```python
from build123d import *

# Parameters (mm, degrees)
SKETCH1_R                = 95.705
BOSS_EXTRUDE1_DEPTH      = 5
SKETCH2_W                = 15
SKETCH2_H                = 9.705675634
BOSS_EXTRUDE2_DEPTH      = 120
SKETCH3_R                = 95.705
SKETCH3_R_2              = 85.705
BOSS_EXTRUDE3_DEPTH      = 10
BOSS_EXTRUDE4_DEPTH      = 14.5
BOSS_EXTRUDE4_DEPTH_BACK = 14.5
SKETCH4_W                = 68.22
SKETCH4_H                = 26.18
SKETCH5_W                = 55
SKETCH5_H                = 20.8
CUT_EXTRUDE1_DEPTH       = 22.77
SKETCH6_W                = 40
SKETCH6_H                = 20.8
CUT_EXTRUDE2_DEPTH       = 5.77
SKETCH8_R                = 2.5
CUT_EXTRUDE3_DEPTH       = 5.77


with BuildPart() as part:
    # Sketch1 → Boss-Extrude1 (new body)
    with BuildSketch(Plane(origin=(0, 0, 0), x_dir=(1, 0, 0), z_dir=(0, 1, 0))):
        with Locations(Location((0, 0, 0), (0, 0, 94.494638706))):
            Circle(SKETCH1_R)
    extrude(amount=BOSS_EXTRUDE1_DEPTH)

    # Sketch2 → Boss-Extrude2 (add)
    with BuildSketch(Plane(origin=(0, 5, 0), x_dir=(1, 0, 0), z_dir=(0, 1, 0))):
        Polygon((83.827926187, 19.351377631), (93.058572244, 22.350596344), (88.423317328, 36.616444088), (79.192671271, 33.617225375), align=None)
        with Locations((0, 90.557837817)):
            Rectangle(SKETCH2_W, SKETCH2_H)
        Polygon((44.30850759, -73.745190895), (50.013360591, -81.597247425), (62.148615507, -72.780468641), (56.443762506, -64.928412111), align=None)
        Polygon((-56.443762506, -64.928412111), (-62.148615507, -72.780468641), (-50.013360591, -81.597247425), (-44.30850759, -73.745190895), align=None)
        Polygon((-79.192671271, 33.617225375), (-88.423317328, 36.616444088), (-93.058572244, 22.350596344), (-83.827926187, 19.351377631), align=None)
    extrude(amount=BOSS_EXTRUDE2_DEPTH)

    # Sketch3 → Boss-Extrude3 (add)
    with BuildSketch(Plane(origin=(0, 125, 0), x_dir=(1, 0, 0), z_dir=(0, 1, 0))):
        with Locations(Location((0, 0, 0), (0, 0, 94.494638706))):
            Circle(SKETCH3_R)
        Circle(SKETCH3_R_2, mode=Mode.SUBTRACT)
    extrude(amount=BOSS_EXTRUDE3_DEPTH)

    # Sketch4 → Boss-Extrude4 (add, two sides: drawn at the far end of the back side and taken through both)
    with BuildSketch(Plane(origin=(0, 130, 0), x_dir=(1, 0, 0), z_dir=(0, 1, 0)).offset(-BOSS_EXTRUDE4_DEPTH_BACK)):
        with Locations((-13.22, 84.54)):
            Rectangle(SKETCH4_W, SKETCH4_H)
    extrude(amount=BOSS_EXTRUDE4_DEPTH + BOSS_EXTRUDE4_DEPTH_BACK)

    # Sketch5 → Cut-Extrude1 (cut)
    with BuildSketch(Plane(origin=(0, 0, -97.63), x_dir=(-1, 0, 0), z_dir=(0, 0, -1))):
        with Locations((10, 130)):
            Rectangle(SKETCH5_W, SKETCH5_H)
    extrude(amount=-CUT_EXTRUDE1_DEPTH, mode=Mode.SUBTRACT)

    # Sketch6 → Cut-Extrude2 (cut)
    with BuildSketch(Plane(origin=(0, 0, -74.86), x_dir=(-1, 0, 0), z_dir=(0, 0, -1))):
        with Locations((10, 130)):
            Rectangle(SKETCH6_W, SKETCH6_H)
    extrude(amount=-CUT_EXTRUDE2_DEPTH, mode=Mode.SUBTRACT)

    # Sketch8 → Cut-Extrude3 (cut)
    with BuildSketch(Plane.XY.offset(90.705)):
        with Locations((0, 130)):
            Circle(SKETCH8_R)
    extrude(amount=-CUT_EXTRUDE3_DEPTH, mode=Mode.SUBTRACT)


solid = part.part
```
The listing builds one solid part. Answer for the finished solid, in the listing's coordinates (mm). A direction names the side the tool comes from. Round coordinates to 2 decimals unless told otherwise and drop trailing zeros. Write each loop counter-clockwise with the first axis right and the second up, starting at its lowest first coordinate (ties: lowest second). Pieces come first, ordered by that corner, then holes. Notation, with made-up numbers: (46.5, -24) -> (58.5, -24) arc R21 ccw to (58.5, 2) -> close; hole circle Ø1 at (10, 44). An arc over 180 degrees is marked (long way). Use CSV: the item, a comma, the result in double quotes. Start each with the question number.
(1) Which of the six approach directions +Z, -Z, +X, -X, +Y, -Y give full straight-line access (tool end or side, diameter ignored) to faces 1 (the face through (14, 130, -74.86)), 2 (the face through (0, 59, -85.705)), 3 (the face through (-7.5, 59, -90)), 4 (the face through (81.48, 64.16, -26.58)), 5 (the face through (88.38, 64.16, -20.83))?
(2) Section C-C on z = 0 is taken. Give the vertices of the cut face in (x, y) (3 decimals).
(3) Consider L1, parallel to X at y = 129, z = 0 (3 decimals); L2, parallel to Y at x = -80, z = -48; L3, parallel to Y at x = -18, z = 31.5. Determine where each line is inside the solid, lowest interval first. Write a range as from..to.
(4) Each of these flat-tipped pins is pushed along its axis until it touches: pin 1 (10.5 mm diameter, centred on y = 60.5, z = -91.5, fed in from -X); pin 2 (12 mm diameter, centred on x = 0, y = 85.5, fed in from +Z) (3 decimals); pin 3 (12 mm diameter, centred on x = -3, y = 74.5, fed in from -Z). Where does it stop, or does it pass through?
(5) Section B-B on y = 108.5 is taken. Give the vertices of the cut face in (x, z) (1 decimal), then the cut area to 3 significant figures.
(6) The mould has two halves that part along X. Classify faces 6 (the face through (90.773, 64.16, -29.384)), 7 (the face through (-58.955, 2.465, 75.39)), 8 (the face through (-47.201, 64.16, 77.726)): released by +X, released by -X, zero draft, split by the parting line, or undercut.
(7) Section A-A on x = 0 is taken. Give the vertices of the cut face in (y, z) (3 decimals).
A:
1,face 1,"-Z"
1,face 2,"+Z, +X, -X"
1,face 3,"+Z, -Z, -X"
1,face 4,"+Z"
1,face 5,"+Z, +X"
2,outline,"(-95.705, 0) -> (95.705, 0) -> (95.705, 5) -> (-95.705, 5) -> close; (-95.705, 125) -> (-85.705, 125) -> (-85.705, 135) -> (-95.705, 135) -> close; (85.705, 125) -> (95.705, 125) -> (95.705, 135) -> (85.705, 135) -> close"
3,L1,"x = -95.705..-85.705, 85.705..95.705"
3,L2,"y = 0..5, 125..135"
3,L3,"y = 0..5"
4,pin 1,"stops at x = -7.5"
4,pin 2,"stops at z = -85.705"
4,pin 3,"stops at z = -95.41"
5,outline,"(-93.1, -22.4) -> (-88.4, -36.6) -> (-79.2, -33.6) -> (-83.8, -19.4) -> close; (-62.1, 72.8) -> (-56.4, 64.9) -> (-44.3, 73.7) -> (-50, 81.6) -> close; (-7.5, -95.4) -> (7.5, -95.4) -> (7.5, -85.7) -> (-7.5, -85.7) -> close; (44.3, 73.7) -> (56.4, 64.9) -> (62.1, 72.8) -> (50, 81.6) -> close; (79.2, -33.6) -> (88.4, -36.6) -> (93.1, -22.4) -> (83.8, -19.4) -> close"
5,area,"728 mm²"
6,face 6,"released by +X"
6,face 7,"split by the parting line"
6,face 8,"undercut"
7,outline,"(0, -95.705) -> (5, -95.705) -> (5, -95.411) -> (115.5, -95.411) -> (115.5, -97.63) -> (119.6, -97.63) -> (119.6, -71.45) -> (115.5, -71.45) -> (115.5, -85.705) -> (5, -85.705) -> (5, 95.705) -> (0, 95.705) -> close; (125, 85.705) -> (127.5, 85.705) -> (127.5, 90.705) -> (132.5, 90.705) -> (132.5, 85.705) -> (135, 85.705) -> (135, 95.705) -> (125, 95.705) -> close; (140.4, -97.63) -> (144.5, -97.63) -> (144.5, -71.45) -> (140.4, -71.45) -> close"
